```python
from build123d import *

# Parameters (mm, degrees)
SKETCH4_W               = 42
SKETCH4_H               = 42
BOTTOM_DEPTH            = 9.4
CHAMFER2_SIZE           = 5
SKETCH6_W               = 42
SKETCH6_H               = 42
MIDDLE_DEPTH            = 28.2
CHAMFER3_SIZE           = 7
SKETCH8_W               = 42
SKETCH8_H               = 42
TOP_DEPTH               = 9.4
CHAMFER4_SIZE           = 5
SKETCH9_R               = 11
SKETCH9_R_2             = 3.5
BOSS_EXTRUDE4_DEPTH     = 2
SKETCH10_R              = 2.5
SHAFT_DEPTH             = 24
CUT_EXTRUDE3_DEPTH      = 5
CUT_EXTRUDE3_DEPTH_BACK = 5
SKETCH11_W              = 2.239647547
SKETCH11_H              = 11.242457261


with BuildPart() as part:
    # Sketch4 → Bottom (new body)
    with BuildSketch(Plane(origin=(0, 0, 0), x_dir=(1, 0, 0), z_dir=(0, 1, 0))):
        Rectangle(SKETCH4_W, SKETCH4_H)
    extrude(amount=BOTTOM_DEPTH)

    # Chamfer2
    chamfer2_edges = [part.edges().sort_by_distance(p)[0] for p in [
        (-21, 4.7, 21),
        (-21, 4.7, -21),
        (21, 4.7, -21),
        (21, 4.7, 21),
    ]]
    chamfer(chamfer2_edges, length=CHAMFER2_SIZE)

    # Sketch6 → Middle (add)
    with BuildSketch(Plane(origin=(0, 9.4, 0), x_dir=(1, 0, 0), z_dir=(0, 1, 0))):
        Rectangle(SKETCH6_W, SKETCH6_H)
    extrude(amount=MIDDLE_DEPTH)

    # Chamfer3
    chamfer3_edges = [part.edges().sort_by_distance(p)[0] for p in [
        (21, 23.5, 21),
        (-21, 23.5, 21),
        (-21, 23.5, -21),
        (21, 23.5, -21),
    ]]
    chamfer(chamfer3_edges, length=CHAMFER3_SIZE)

    # Sketch8 → Top (add)
    with BuildSketch(Plane(origin=(0, 37.6, 0), x_dir=(1, 0, 0), z_dir=(0, 1, 0))):
        Rectangle(SKETCH8_W, SKETCH8_H)
    extrude(amount=TOP_DEPTH)

    # Chamfer4
    chamfer4_edges = [part.edges().sort_by_distance(p)[0] for p in [
        (21, 42.3, 21),
        (21, 42.3, -21),
        (-21, 42.3, -21),
        (-21, 42.3, 21),
    ]]
    chamfer(chamfer4_edges, length=CHAMFER4_SIZE)

    # Sketch9 → Boss-Extrude4 (add)
    with BuildSketch(Plane(origin=(0, 47, 0), x_dir=(1, 0, 0), z_dir=(0, 1, 0))):
        with Locations(Location((0, 0, 0), (0, 0, 270))):
            Circle(SKETCH9_R)
        with Locations(Location((0, 0, 0), (0, 0, 270))):
            Circle(SKETCH9_R_2, mode=Mode.SUBTRACT)
    extrude(amount=BOSS_EXTRUDE4_DEPTH)

    # Sketch10 → Shaft (add)
    with BuildSketch(Plane(origin=(0, 47, 0), x_dir=(1, 0, 0), z_dir=(0, 1, 0))):
        with Locations(Location((0, 0, 0), (0, 0, 90))):
            Circle(SKETCH10_R)
    extrude(amount=SHAFT_DEPTH)

    # Sketch11 → Cut-Extrude3 (cut, two sides: drawn at the far end of the back side and taken through both)
    with BuildSketch(Plane(origin=(0, 0, 0), x_dir=(0, 0, -1), z_dir=(1, 0, 0)).offset(-CUT_EXTRUDE3_DEPTH_BACK)):
        with Locations((2.338622492, 67.62122863)):
            Rectangle(SKETCH11_W, SKETCH11_H)
    extrude(amount=CUT_EXTRUDE3_DEPTH + CUT_EXTRUDE3_DEPTH_BACK, mode=Mode.SUBTRACT)


solid = part.part
```
Input: part model. Units: mm. Frame: model coordinates. A direction names the side the tool comes from. Coordinates: 2 decimals unless noted, no trailing zeros. Write each loop counter-clockwise with the first axis right and the second up, starting at its lowest first coordinate (ties: lowest second). Pieces come first, ordered by that corner, then holes. Notation, with made-up numbers: (88.25, -21) -> (109.25, -21) arc R38 cw to (109.25, 18) -> close; hole circle Ø3 at (-38, -8). An arc over 180 degrees is marked (long way). Answer as a JSON object with one key per item and string values.
1. Section D-D on z = 0. Return the cut outline in (x, y), then the cut area to 3 significant figures.
Result set:
{"outline": "(-21, 0) -> (21, 0) -> (21, 47) -> (11, 47) -> (11, 49) -> (3.5, 49) -> (3.5, 47) -> (2.5, 47) -> (2.5, 71) -> (-2.5, 71) -> (-2.5, 47) -> (-3.5, 47) -> (-3.5, 49) -> (-11, 49) -> (-11, 47) -> (-21, 47) -> close", "area": "2,120 mm2"}
2. Section A-A on z = 15. Return the cut outline in (x, y), then the cut area to 3 significant figures.
Result set:
{"outline": "(-21, 37.6) -> (-20, 37.6) -> (-20, 0) -> (20, 0) -> (20, 37.6) -> (21, 37.6) -> (21, 47) -> (-21, 47) -> close", "area": "1,900 mm2"}
3. Section B-B on y = 43.5. Return the cut outline in (x, z).
Result set:
{"outline": "(-21, -16) -> (-16, -21) -> (16, -21) -> (21, -16) -> (21, 16) -> (16, 21) -> (-16, 21) -> (-21, 16) -> close"}
4. Mould query, pull axis X, two halves, no side actions, for faces 4 (the face through (-3.417, 47.986, -0.759)), 5 (the face through (3, 49, -3)), 6 (the face through (-17, 19, -18)), 7 (the face through (19, 42, -18)). Classes: released by +X, released by -X, zero draft, split by the parting line, or undercut.
Result set:
{"face 4": "undercut", "face 5": "zero draft", "face 6": "released by -X", "face 7": "released by +X"}
5. Access query for faces 1 (the face through (-17, 19, 18)), 2 (the face through (1.5, 58.8, 2)), 3 (the face through (18, 19, -17)). Directions: +Z, -Z, +X, -X, +Y, -Y. A direction counts if a zero-diameter tool reaches every point of the face in a straight line with its end or side. Return the directions, or none.
Result set:
{"face 1": "+Z, -X, -Y", "face 2": "+Y", "face 3": "-Z, +X, -Y"}
6. First-contact query: P1, Ø2, axis at x = 18, z = -18.5, coming from the -Y side; P2, Ø21, axis at x = -5, z = 10, coming from the +Y side; P3, Ø0.6, axis at x = -0.5, z = -2, coming from the +Y side; P4, Ø8, axis at x = 1, z = 14, coming from the +Y side. Flat tips, straight axial feed; report the tip coordinate or a pass-through.
Result set:
{"P1": "stops at y = 37.6", "P2": "stops at y = 71", "P3": "stops at y = 62", "P4": "stops at y = 49"}
7. Section C-C on x = 0. Return the cut outline in (y, z), then the cut area to 3 significant figures.
Result set:
{"outline": "(0, -21) -> (47, -21) -> (47, -11) -> (49, -11) -> (49, -3.5) -> (47, -3.5) -> (47, -2.5) -> (62, -2.5) -> (62, -1.22) -> (71, -1.22) -> (71, 2.5) -> (47, 2.5) -> (47, 3.5) -> (49, 3.5) -> (49, 11) -> (47, 11) -> (47, 21) -> (0, 21) -> close", "area": "2,110 mm2"}
8. Material intervals for line 1 (X direction, y = 47.9, z = 0); line 2 (Y direction, x = 5, z = -7.5); line 3 (Y direction, x = 16.5, z = 16.5), sorted ascending. Write a range as from..to.
Result set:
{"line 1": "x = -11..-3.5, -2.5..2.5, 3.5..11", "line 2": "y = 0..49", "line 3": "y = 0..47"}
